from build123d import *

# Parameters (mm, degrees)
ESQUISSE1_W                  = 50
ESQUISSE1_H                  = 410
BOSS_EXTRU_1_DEPTH           = 15
ENL_V_MAT_EXTRU_1_DEPTH      = 414.309811159
ENL_V_MAT_EXTRU_1_DEPTH_BACK = 414.309811159
ESQUISSE2_R                  = 5
ESQUISSE2_R_2                = 2.25
CONG_1_R                     = 10


with BuildPart() as part:
    # Esquisse1 → Boss.-Extru.1 (new body)
    with BuildSketch(Plane.XY):
        with Locations((25, 205)):
            Rectangle(ESQUISSE1_W, ESQUISSE1_H)
    extrude(amount=BOSS_EXTRU_1_DEPTH)

    # Esquisse2 → Enlèv. mat.-Extru.1 (cut, two sides: drawn at the far end of the back side and taken through both)
    with BuildSketch(Plane.XY.offset(15).offset(-ENL_V_MAT_EXTRU_1_DEPTH_BACK)):
        with Locations((25, 240.5)):
            Circle(ESQUISSE2_R)
        with Locations((25, 311.5)):
            Circle(ESQUISSE2_R)
        with Locations((25, 382.5)):
            Circle(ESQUISSE2_R)
        with Locations(Location((25, 27.5, 0), (0, 0, 180))):
            Circle(ESQUISSE2_R)
        with Locations(Location((25, 98.5, 0), (0, 0, 180))):
            Circle(ESQUISSE2_R)
        with Locations(Location((25, 169.5, 0), (0, 0, 180))):
            Circle(ESQUISSE2_R)
        with Locations((40, 271)):
            Circle(ESQUISSE2_R_2)
        with Locations((40, 403)):
            Circle(ESQUISSE2_R_2)
        with Locations(Location((40, 7, 0), (0, 0, 180))):
            Circle(ESQUISSE2_R_2)
        with Locations(Location((40, 139, 0), (0, 0, 180))):
            Circle(ESQUISSE2_R_2)
        with Locations((10, 139)):
            Circle(ESQUISSE2_R_2)
        with Locations((10, 7)):
            Circle(ESQUISSE2_R_2)
        with Locations(Location((10, 403, 0), (0, 0, 180))):
            Circle(ESQUISSE2_R_2)
        with Locations(Location((10, 271, 0), (0, 0, 180))):
            Circle(ESQUISSE2_R_2)
    extrude(amount=ENL_V_MAT_EXTRU_1_DEPTH + ENL_V_MAT_EXTRU_1_DEPTH_BACK, mode=Mode.SUBTRACT)

    # Congé1
    cong_1_edges = [part.edges().sort_by_distance(p)[0] for p in [
        (0, 410, 7.5),
        (50, 410, 7.5),
        (50, 0, 7.5),
        (0, 0, 7.5),
    ]]
    fillet(cong_1_edges, radius=CONG_1_R)


solid = part.part
Source: CAD feature listing. Evaluate the final solid. Frame: model axes, mm. Round coordinates to 2 decimals unless told otherwise and drop trailing zeros. Loops run counter-clockwise (first coordinate to the right, second up) from the corner with the lowest first, then second, coordinate; pieces in that order, holes last. Notation, with made-up numbers: (37.25, 89) - (57.25, 89) arc R23 ccw to (57.25, 110) - close; hole circle Ø4 at (-27.75, -36). An arc over 180 degrees is marked (long way). Write item = value, one per line. Start each with the question number.
Item 1: Section query B-B on z = 12. Count the separate pieces of the cut face and the enclosed holes in it, plus the area to 3 significant figures.
Item 2: First-contact query: pin 1 Ø5 at (x, y) = (40, 7) entering from +Z. Flat tip, straight axial feed; report the tip coordinate or a pass-through.
Item 3: Section query A-A on y = 98.5. Output: boundary loops of the cut face in (x, z), plus the area to 3 significant figures.
Item 4: Material intervals for line 1 (X direction, y = 271, z = 10.75); line 2 (Y direction, x = 40, z = 3.25); line 3 (X direction, y = 240.5, z = 5.75), sorted ascending.
Item 5: Mould query, pull axis X, two halves, no side actions, for faces 1 (the face through (29.995, 169.28, 7.395)), 2 (the face through (25, 208, 15)), 3 (the face through (2.85, 3.01, 7.6)), 4 (the face through (50, 202, 7)). Classes: released by +X, released by -X, zero draft, split by the parting line, or undercut.
Results list:
q1.separate_pieces = 1
q1.enclosed_holes = 14
q1.area = 19,800 mm²
q2.pin_1 = 15
q3.outline = (0, 0) - (20, 0) - (20, 15) - (0, 15) - close; (30, 0) - (50, 0) - (50, 15) - (30, 15) - close
q3.area = 600 mm²
q4.line_1 = 0 to 7.75, 12.25 to 37.75, 42.25 to 50
q4.line_2 = 0 to 4.75, 9.25 to 136.75, 141.25 to 268.75, 273.25 to 400.75, 405.25 to 410
q4.line_3 = 0 to 20, 30 to 50
q5.face_1 = undercut
q5.face_2 = zero draft
q5.face_3 = released by -X
q5.face_4 = released by +X
